```python
from build123d import *

# Parameters (mm, degrees)
SKETCH1_R           = 2.5
SKETCH1_R_2         = 1.5
BOSS_EXTRUDE1_DEPTH = 3


with BuildPart() as part:
    # Sketch1 → Boss-Extrude1 (new body)
    with BuildSketch(Plane.XY):
        with BuildLine():
            Line((-28, -47.5), (28, -47.5))
            ThreePointArc((28, -47.5), (29.414213562, -46.914213562), (30, -45.5))
            Line((30, -45.5), (30, 45.5))
            ThreePointArc((30, 45.5), (29.414213562, 46.914213562), (28, 47.5))
            Line((28, 47.5), (-28, 47.5))
            ThreePointArc((-28, 47.5), (-29.414213562, 46.914213562), (-30, 45.5))
            Line((-30, 45.5), (-30, -45.5))
            ThreePointArc((-30, -45.5), (-29.414213562, -46.914213562), (-28, -47.5))
        make_face()
        with Locations((0, 37.5)):
            Circle(SKETCH1_R, mode=Mode.SUBTRACT)
        with Locations((0, -37.5)):
            Circle(SKETCH1_R, mode=Mode.SUBTRACT)
        with Locations((-15, 24.5)):
            Circle(SKETCH1_R_2, mode=Mode.SUBTRACT)
        with Locations((15, 24.5)):
            Circle(SKETCH1_R_2, mode=Mode.SUBTRACT)
        with Locations((-15, -8.5)):
            Circle(SKETCH1_R_2, mode=Mode.SUBTRACT)
        with Locations((15, -8.5)):
            Circle(SKETCH1_R_2, mode=Mode.SUBTRACT)
        with BuildLine():
            Line((-11.5, -9.5), (-11.5, -6.5))
            ThreePointArc((-11.5, -6.5), (-12.085786438, -5.085786438), (-13.5, -4.5))
            Line((-13.5, -4.5), (-16.5, -4.5))
            ThreePointArc((-16.5, -4.5), (-17.914213562, -3.914213562), (-18.5, -2.5))
            Line((-18.5, -2.5), (-18.5, 3.5))
            ThreePointArc((-18.5, 3.5), (-17.914213562, 4.914213562), (-16.5, 5.5))
            Line((-16.5, 5.5), (16.5, 5.5))
            ThreePointArc((16.5, 5.5), (17.914213562, 4.914213562), (18.5, 3.5))
            Line((18.5, 3.5), (18.5, -2.5))
            ThreePointArc((18.5, -2.5), (17.914213562, -3.914213562), (16.5, -4.5))
            Line((16.5, -4.5), (13.5, -4.5))
            ThreePointArc((13.5, -4.5), (12.085786438, -5.085786438), (11.5, -6.5))
            Line((11.5, -6.5), (11.5, -9.5))
            ThreePointArc((11.5, -9.5), (10.914213562, -10.914213562), (9.5, -11.5))
            Line((9.5, -11.5), (-9.5, -11.5))
            ThreePointArc((-9.5, -11.5), (-10.914213562, -10.914213562), (-11.5, -9.5))
        make_face(mode=Mode.SUBTRACT)
    extrude(amount=BOSS_EXTRUDE1_DEPTH)


solid = part.part
```
Design review of the part built by this model. Coordinates are the model's own, in mm. A direction names the side the tool comes from. Round coordinates to 2 decimals unless told otherwise and drop trailing zeros. Order: outer loops, then holes, each group sorted by start corner. A loop starts at its lowest first (then second) coordinate and runs counter-clockwise, first axis right, second up. Notation, with made-up numbers: (-2.75, -21) - (37.25, -21) arc R24 cw to (37.25, -8) - close; hole circle Ø6 at (13.5, -18). An arc over 180 degrees is marked (long way). Return JSON: item names as keys, results as strings.
Q1. Consider section A-A on y = 24.5. Write out the cut boundary in (x, z).
Computed values:
{"outline": "(-30, 0) - (-16.5, 0) - (-16.5, 3) - (-30, 3) - close; (-13.5, 0) - (13.5, 0) - (13.5, 3) - (-13.5, 3) - close; (16.5, 0) - (30, 0) - (30, 3) - (16.5, 3) - close"}
Q2. Consider section C-C on x = 1.5. Write out the cut boundary in (y, z), plus the area to 3 significant figures.
Computed values:
{"outline": "(-47.5, 0) - (-39.5, 0) - (-39.5, 3) - (-47.5, 3) - close; (-35.5, 0) - (-11.5, 0) - (-11.5, 3) - (-35.5, 3) - close; (5.5, 0) - (35.5, 0) - (35.5, 3) - (5.5, 3) - close; (39.5, 0) - (47.5, 0) - (47.5, 3) - (39.5, 3) - close", "area": "210 mm2"}
Q3. The part is to be moulded in two halves that separate along Y. For faces 3 (the cylindrical face through (29.4, -46.93, 1.48)), 4 (the flat face through (0, 11, 3)), 5 (the flat face through (-15, -4.5, 1)), say which applies: pulls with the +Y half, pulls with the -Y half, needs draft (parallel to the pull), parting line crosses it, or undercut.
Computed values:
{"face 3": "pulls with the -Y half", "face 4": "needs draft", "face 5": "undercut"}
Q4. For pin 1 Ø2.5 at (x, y) = (-15, -8.5) entering from +Z, flat-tipped, find the tip position at first contact; note if it passes through.
Computed values:
{"pin 1": "passes through"}
Q5. Consider section D-D on y = -8.5. Write out the cut boundary in (x, z), plus the area to 3 significant figures.
Computed values:
{"outline": "(-30, 0) - (-16.5, 0) - (-16.5, 3) - (-30, 3) - close; (-13.5, 0) - (-11.5, 0) - (-11.5, 3) - (-13.5, 3) - close; (11.5, 0) - (13.5, 0) - (13.5, 3) - (11.5, 3) - close; (16.5, 0) - (30, 0) - (30, 3) - (16.5, 3) - close", "area": "93.0 mm2"}
Q6. Wall thickness on L1, parallel to Y at x = 0, z = 1.6; L2, parallel to Y at x = 15, z = 1; L3, parallel to Y at x = -5, z = 0.8: over which ranges is each line inside the solid? List them lowest first. Write a range as [from, to].
Computed values:
{"L1": "y = [-47.5, -40], [-35, -11.5], [5.5, 35], [40, 47.5]", "L2": "y = [-47.5, -10], [-7, -4.5], [5.5, 23], [26, 47.5]", "L3": "y = [-47.5, -11.5], [5.5, 47.5]"}
Q7. Consider section B-B on z = 1.2. Give the number of separate pieces and of enclosed holes in the cut face, plus the area to 3 significant figures.
Computed values:
{"separate pieces": "1", "enclosed holes": "7", "area": "5,100 mm2"}
Q8. Machinability: for faces 1 (the flat face through (-18.5, 0, 1)), 2 (the cylindrical face through (29.43, 46.9, 1.48)), which of the approach directions +Z, -Z, +X, -X, +Y, -Y give a long, thin tool a straight path to every point of the face, cutting with its end or side? Answer none if there is none.
Computed values:
{"face 1": "+Z, -Z", "face 2": "+Z, -Z, +X, +Y"}
